from build123d import *

# Parameters (mm, degrees)
SKETCH_1_W                  = 11
SKETCH_1_H                  = 3
EXTRUDE_1_DEPTH             = 13
HOLE_WIZARD_2_5_2_5_1_D     = 2.5
HOLE_WIZARD_2_5_2_5_1_DEPTH = 16
HOLE_WIZARD_3_2_3_2_1_D     = 3.2
HOLE_WIZARD_3_2_3_2_1_DEPTH = 16
HOLE_WIZARD_6_0_6_1_D       = 6
HOLE_WIZARD_3_2_3_2_2_D     = 3.2
HOLE_WIZARD_3_2_3_2_2_DEPTH = 16


with BuildPart() as part:
    # 草图1 → 旋转1 (revolve)
    with BuildSketch(Plane.XZ, mode=Mode.PRIVATE) as revolve_1_sk:
        with Locations((5.5, 1.5)):
            Rectangle(SKETCH_1_W, SKETCH_1_H)
    revolve(revolve_1_sk.sketch.rotate(Axis((0, 0, 3), (0, 0, -1)), 180), axis=Axis((0, 0, 3), (0, 0, -1)))

    # 草图2 → 凸台-拉伸1 (add)
    with BuildSketch(Plane.XY.offset(3)):
        with BuildLine():
            Line((7.483314774, -5), (-7.907139717, -5))
            ThreePointArc((-7.907139717, -5), (-9.257527395, -1.630006909), (-9.198789331, 2))
            Line((-9.198789331, 2), (8.774964387, 2))
            ThreePointArc((8.774964387, 2), (8.833702451, -1.630006909), (7.483314774, -5))
        make_face()
    extrude(amount=EXTRUDE_1_DEPTH)

    # Ø2.5 (2.5) 直径孔1
    with Locations(Plane(origin=(0, 0, 0), x_dir=(-1, 0, 0), z_dir=(0, 0, -1))):
        with Locations((0, -7), (0, 7)):
            Hole(HOLE_WIZARD_2_5_2_5_1_D / 2, depth=HOLE_WIZARD_2_5_2_5_1_DEPTH)

    # Ø3.2 (3.2) 直径孔1
    with Locations(Plane(origin=(0, -5, 0), x_dir=(-1, 0, 0), z_dir=(0, -1, 0))):
        with Locations((5, -8), (-5, -8)):
            Hole(HOLE_WIZARD_3_2_3_2_1_D / 2, depth=HOLE_WIZARD_3_2_3_2_1_DEPTH)

    # Ø6.0 (6) 直径孔1 (through all)
    with Locations(Plane(origin=(0, 0, 0), x_dir=(-1, 0, 0), z_dir=(0, 0, -1))):
        with Locations((0, 0)):
            Hole(HOLE_WIZARD_6_0_6_1_D / 2)

    # Ø3.2 (3.2) 直径孔2
    with Locations(Plane(origin=(0, -5, 0), x_dir=(-1, 0, 0), z_dir=(0, -1, 0))):
        with Locations((0, -14)):
            Hole(HOLE_WIZARD_3_2_3_2_2_D / 2, depth=HOLE_WIZARD_3_2_3_2_2_DEPTH)


solid = part.part
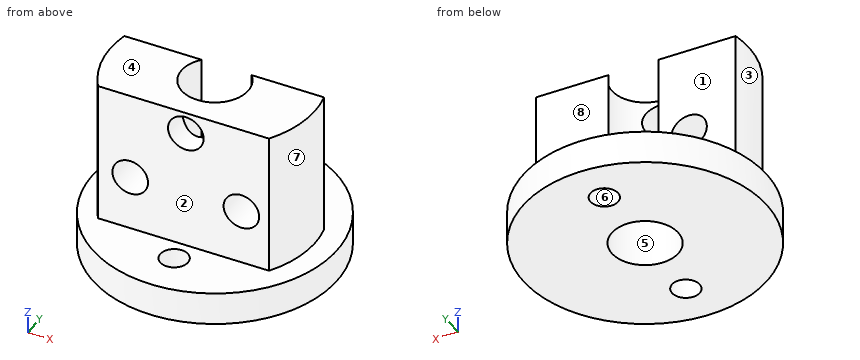
Could you check a few things on this model? Use its own coordinates, in mm. Face numbers are marked on the shaded views. A direction names the side the tool comes from. Coordinates: 2 decimals unless noted, no trailing zeros. Write each loop counter-clockwise with the first axis right and the second up, starting at its lowest first coordinate (ties: lowest second). Pieces come first, ordered by that corner, then holes. Notation, with made-up numbers: (83, 87) - (138, 87) arc R25 ccw to (138, 99) - close; hole circle Ø7 at (25.5, 76.25). An arc over 180 degrees is marked (long way). Put each result on its own line as item: value. Start each with the question number.
Q1. Thinking about a two-plate mould opening in Y: for the marked faces 5, 6, 7 and 8, which applies, pulls with the +Y half, pulls with the -Y half, needs draft (parallel to the pull), parting line crosses it, or undercut?
Q2. Which directions (+Z, -Z, +X, -X, +Y, -Y) give clear straight access to the entire face, cutting with the end or side of a thin tool? Please do the marked faces 1, 2, 3 and 4.
Q3. I want a section at D-D on z = 5.5. Write out the boundary of the cut face in (x, y), plus the area to 3 significant figures.
Q4. I want a section at A-A on z = 14. Write out the boundary of the cut face in (x, y).
Q5. I want a section at C-C on y = 7. Write out the boundary of the cut face in (x, z), plus the area to 3 significant figures.
Q6. Please list where these lines run through material, in increasing order: L1, parallel to Y at x = 0, z = 1.4; L2, parallel to Z at x = 0, y = -4.1; L3, parallel to Z at x = 5, y = -2.25.
Q7. I want a section at B-B on x = 4.75. Write out the boundary of the cut face in (y, z).
Q8. I'm going to push flat-ended pins straight in: P1, Ø3.5, axis at x = 6.5, z = 11.5, coming from the +Y side; P2, Ø1.5, axis at x = 0.5, y = -8, coming from the +Z side; P3, Ø4, axis at x = 0, z = 14, coming from the +Y side. Where does each tip first touch, or does it pass through?
Checks:
1. face 5: undercut
1. face 6: undercut
1. face 7: parting line crosses it
1. face 8: pulls with the +Y half
2. face 1: +Z, +X, -X, +Y
2. face 2: +Z, +X, -X, -Y
2. face 3: +Z, -X
2. face 4: +Z, +X, -X, +Y, -Y
3. outline: (-9.2, 2) arc R9.2 ccw to (-7.91, -5) - (7.48, -5) arc R9.2 ccw to (8.77, 2) - (2.24, 2) arc R3 cw (long way) to (-2.24, 2) - close
3. area: 98.5 mm²
4. outline: (-9.2, 2) arc R9.2 ccw to (-7.91, -5) - (-1.6, -5) - (-1.6, -2.54) arc R3 cw to (-2.24, 2) - close; (1.6, -5) - (7.48, -5) arc R9.2 ccw to (8.77, 2) - (2.24, 2) arc R3 cw to (1.6, -2.54) - close
5. outline: (-8.49, 0) - (-1.25, 0) - (-1.25, 3) - (-8.49, 3) - close; (1.25, 0) - (8.49, 0) - (8.49, 3) - (1.25, 3) - close
5. area: 43.4 mm²
6. L1: -11 to -8.25, -5.75 to -3, 3 to 5.75, 8.25 to 11
6. L2: 0 to 12.4, 15.6 to 16
6. L3: 0 to 6.4, 9.6 to 16
7. outline: (-9.92, 0) - (9.92, 0) - (9.92, 3) - (2, 3) - (2, 6.42) - (-5, 6.42) - (-5, 3) - (-9.92, 3) - close; (-5, 9.58) - (2, 9.58) - (2, 16) - (-5, 16) - close
8. P1: y = 2
8. P2: z = 3
8. P3: y = -2.24
